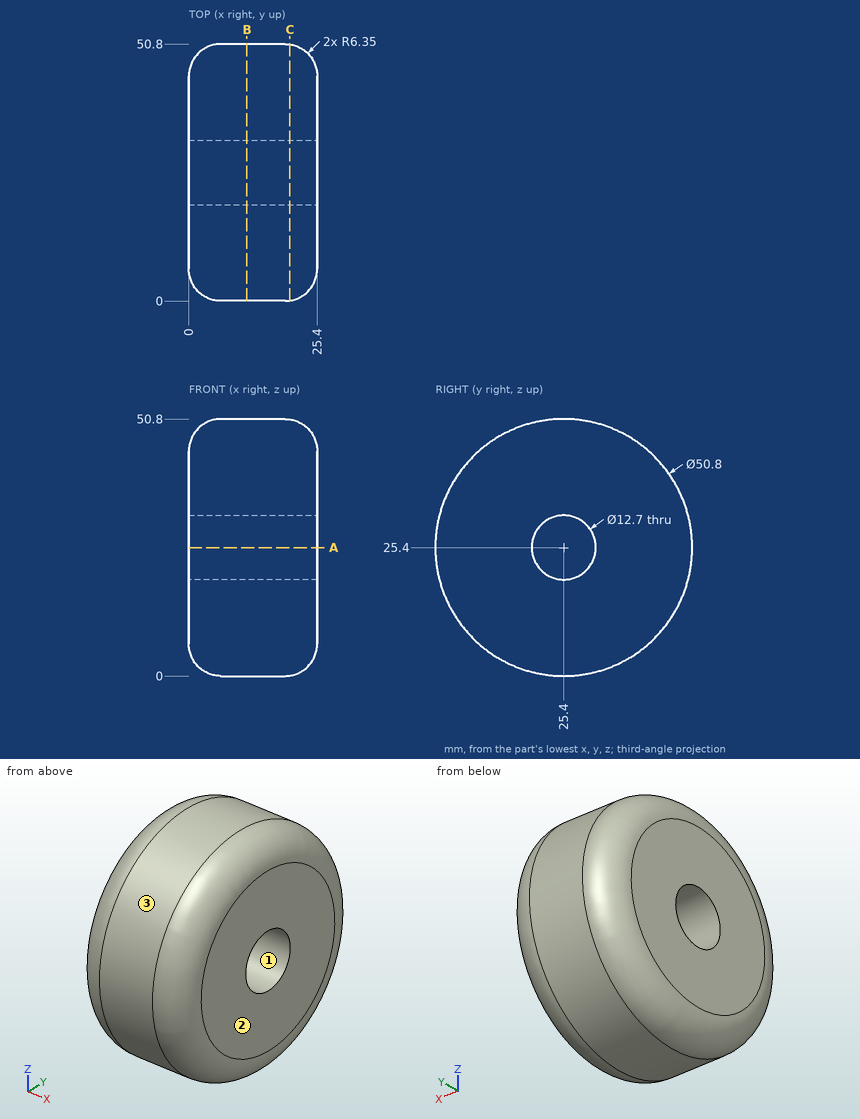
Source: three-view drawing plus pictorial views. Frame: mm from the lowest corner of the part. Coordinates: 2 decimals unless noted, no trailing zeros. Loops run counter-clockwise (first coordinate to the right, second up) from the corner with the lowest first, then second, coordinate; pieces in that order, holes last. Notation, with made-up numbers: M 8,-5 L 54,-5 A18 cw 54,23 Z; hole C 50,15.5 d11. An arc over 180 degrees is marked long. Use CSV: the item, a comma, the result in double quotes.
(1) Cut plane A-A on z = 25.4. Return loops of the section in (x, y).
Answers follow:
outline,"M 0,6.35 A6.35 ccw 6.35,0 L 19.05,0 A6.35 ccw 25.4,6.35 L 25.4,19.05 L 0,19.05 Z; M 0,31.75 L 25.4,31.75 L 25.4,44.45 A6.35 ccw 19.05,50.8 L 6.35,50.8 A6.35 ccw 0,44.45 Z"
(2) Line query: line 1 (Y direction, x = 8.75, z = 25.4); line 2 (X direction, y = 28, z = 44.5); line 3 (Z direction, x = 12.25, y = 24.5). Output: solid intervals per line, ascending. Write a range as [from, to].
Answers follow:
line 1,"[0, 19.05], [31.75, 50.8]"
line 2,"[0, 25.4]"
line 3,"[0.02, 19.11], [31.69, 50.78]"
(3) Contact query for flat-ended pins moving along their axis: pin 1 (8 mm diameter, centred on x = 16, y = 8.5, fed in from +Z); pin 2 (1.5 mm diameter, centred on x = 3.5, z = 43, fed in from -Y); pin 3 (20.5 mm diameter, centred on y = 25.4, z = 25.4, fed in from +X); pin 4 (10 mm diameter, centred on x = 22, y = 18, fed in from -Z). Output: stop coordinate, or through.
Answers follow:
pin 1,"z = 47.28"
pin 2,"y = 7.16"
pin 3,"x = 25.4"
pin 4,"z = 0.2"
(4) Cut plane C-C on x = 20. Return loops of the section in (y, z).
Answers follow:
outline,"C 25.4,25.4 d50.66; hole C 25.4,25.4 d12.7"
(5) Cut plane B-B on x = 11.5. Return loops of the section in (y, z).
Answers follow:
outline,"C 25.4,25.4 d50.8; hole C 25.4,25.4 d12.7"
(6) Draft query along Z for the marked faces 1, 2 and 3. Return one class per face: pulls with the +Z half, pulls with the -Z half, needs draft (parallel to the pull), parting line crosses it, or undercut.
Answers follow:
face 1,"undercut"
face 2,"needs draft"
face 3,"parting line crosses it"
